Geometry check sheet. Reference: the model listing, model coordinates, mm. A direction names the side the tool comes from. Round coordinates to 2 decimals unless told otherwise and drop trailing zeros. Write each loop counter-clockwise with the first axis right and the second up, starting at its lowest first coordinate (ties: lowest second). Pieces come first, ordered by that corner, then holes. Notation, with made-up numbers: M 87.25,76.25 L 145.25,76.25 A31 cw 145.25,109.25 Z; hole C 66.5,11 d2. An arc over 180 degrees is marked long. Put each result on its own line as item: value. Start each with the question number.
(1) Section check A-A on y = 3.25. Record the cut outline in (x, z), then the cut area to 3 significant figures.
(2) Material ranges on probe 1 along X at (y, z) = (2.7, -235); probe 2 along Z at (x, y) = (-140, 2.85); probe 3 along X at (y, z) = (2.25, -120), recorded low to high.
(3) Tool access check on faces 1 (the cylindrical face through (-2.194, 2.028, -47.26)), 2 (the flat face through (-76, 4, -118)). Record the directions out of +Z, -Z, +X, -X, +Y, -Y that give a thin tool (end or side, any length) a straight path to the whole face; none if there is none.
(4) Mould release check, pull along Z, two halves, no side actions. Record for faces 3 (the flat face through (-76, 0, -118)), 4 (the cylindrical face through (-2.315, 2.028, -192.591)): pulls with the +Z half, pulls with the -Z half, needs draft (parallel to the pull), parting line crosses it, or undercut.
Autodesk Inventor part; units mm, degrees
ref_plane "YZ Plane" through (0, 0, 0) normal (1, 0, 0) x (0, 1, 0)
ref_plane "XZ Plane" through (0, 0, 0) normal (0, 1, 0) x (-1, 0, 0)
ref_plane "XY Plane" through (0, 0, 0) normal (0, 0, 1) x (1, 0, 0)
sketch "スケッチ1" plane through (0, 0, 0) normal (0, 1, 0) x (-1, 0, 0)
  line L0 (0, 0) -> (155, 0)
  line L1 (155, 0) -> (155, -240)
  line L2 (155, -240) -> (0, -240)
  line L3 (0, -240) -> (0, 0)
  dimension "d0" = 155
  dimension "d1" = 240
extrude "押し出し1" add sketch "スケッチ1" along normal blind 4
sketch "スケッチ3" plane through (0, 4, 0) normal (0, 1, 0) x (1, 0, 0)
  line L0 (-155, 240) -> (-155, 0)
  line L1 (-155, 0) -> (0, 0)
  line L2 (0, 240) -> (-155, 240)
  point P0 (-150, 5)
  point P1 (-150, 235)
  point P2 (-150, 120)
  point P3 (-155, 120)
  dimension "d11" = 5
  dimension "d12" = 5
  dimension "d13" = 5
  dimension "d14" = 5
  dimension "d15" = 5
  dimension "d16" = 0
hole "穴1" at (-150, 4, -5) at (-150, 4, -235) at (-150, 4, -120) direction (0, -1, 0) diameter 3.5 end through all
sketch "スケッチ5" plane through (0, 0, 0) normal (0, -1, 0) x (1, 0, 0)
  line L0 (0, -90) -> (0, -150) construction
  line L1 (0, 0) -> (0, -240)
  line L2 (-40, -90) -> (-40, -150)
  line L3 (40, -150) -> (40, -90)
  arc A0 (40, -90) -> (-40, -90) centre (0, -90) ccw
  arc A1 (-40, -150) -> (40, -150) centre (0, -150) ccw
  point P0 (0, -120)
  point P1 (0, -190)
  point P2 (0, -50)
  dimension "d17" = 80
  dimension "d18" = 30
extrude "押し出し2" cut sketch "スケッチ5" against normal blind 10 contours L1 A1 L2 A0
sketch "スケッチ6" plane through (0, 0, 0) normal (0, -1, 0) x (1, 0, 0)
  line L0 (0, -240) -> (-155, -240)
  line L1 (0, -190) -> (0, -240)
  line L2 (-155, 0) -> (0, 0)
  line L3 (0, 0) -> (0, -50)
  point P0 (-20, -235)
  point P1 (-140, -235)
  point P2 (-140, -5)
  point P3 (-20, -5)
  dimension "d28" = 120
  dimension "d30" = 20
  dimension "d31" = 5
  dimension "d32" = 5
  dimension "d33" = 120
  dimension "d34" = 5
  dimension "d35" = 20
  dimension "d36" = 5
hole "穴2" at (-20, 0, -235) at (-140, 0, -235) at (-140, 0, -5) at (-20, 0, -5) direction (0, 1, 0) diameter 3.5 end through all
fillet "フィレット1" radius 10 2 edges at (0, 2, -50) (0, 2, -190)
properties part number "slide_panel" material "木材(サクラ)"
Answers follow:
1. outline: M -155,-240 L 0,-240 L 0,-198.99 A10 ccw -8,-189.19 A40 cw -40,-150 L -40,-90 A40 cw -8,-50.81 A10 ccw 0,-41.01 L 0,0 L -155,0 Z; hole C -150,-235 d3.5; hole C -150,-120 d3.5; hole C -150,-5 d3.5; hole C -140,-235 d3.5; hole C -140,-5 d3.5; hole C -20,-235 d3.5; hole C -20,-5 d3.5
1. area: 32,200 mm^2
2. probe 1: x = -155 to -151.75, -148.25 to -141.75, -138.25 to -21.75, -18.25 to 0
2. probe 2: z = -240 to -236.75, -233.25 to -6.75, -3.25 to 0
2. probe 3: x = -155 to -151.75, -148.25 to -40
3. face 1: +X, +Y, -Y
3. face 2: +Z, -Z, +X, -X, +Y
4. face 3: needs draft
4. face 4: undercut
